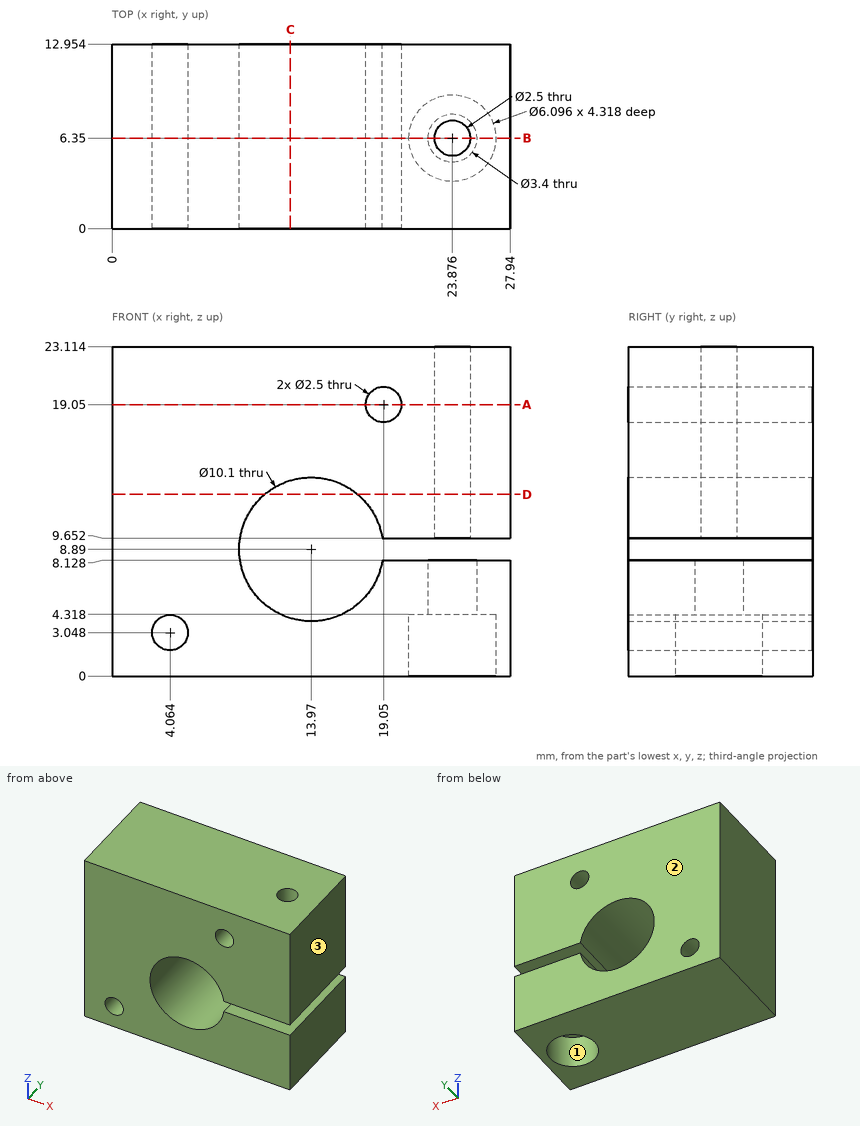
Geometry check sheet. Reference: drawing and pictorial views, mm from the part's lowest x, y, z. Coordinates: 2 decimals unless noted, no trailing zeros. Order: outer loops, then holes, each group sorted by start corner. A loop starts at its lowest first (then second) coordinate and runs counter-clockwise, first axis right, second up.
Item 1: Release check for a two-part mould opening along X. For the marked faces 1, 2 and 3 record: +X half, -X half, draft (parallel to the pull), parting line (faces both ways), or undercut.
Filled in:
face 1: undercut
face 2: draft
face 3: +X half
Item 2: Section check D-D, the plane z = 12.75. Enter the section's corners in (x, y).
Filled in:
outline: (0, 0) - (10.71, 0) - (10.71, 12.95) - (0, 12.95) - close; (17.23, 0) - (27.94, 0) - (27.94, 12.95) - (17.23, 12.95) - close; hole circle Ø2.5 at (23.88, 6.35)
Item 3: Material ranges on L1, parallel to Z at x = 20, y = 7.5; L2, parallel to Z at x = 22.75, y = 9.5; L3, parallel to X at y = 5.5, z = 18.75, recorded low to high.
Filled in:
L1: z = 0 to 8.13, 9.65 to 18.24, 19.86 to 23.11
L2: z = 0 to 8.13, 9.65 to 23.11
L3: x = 0 to 17.84, 20.26 to 22.96, 24.79 to 27.94
Item 4: Section check C-C, the plane x = 12.5. Enter the section's corners in (y, z).
Filled in:
outline: (0, 0) - (12.95, 0) - (12.95, 4.06) - (0, 4.06) - close; (0, 13.72) - (12.95, 13.72) - (12.95, 23.11) - (0, 23.11) - close
Item 5: Section check A-A, the plane z = 19.05. Enter the section's corners in (x, y).
Filled in:
outline: (0, 0) - (17.8, 0) - (17.8, 12.95) - (0, 12.95) - close; (20.3, 0) - (27.94, 0) - (27.94, 12.95) - (20.3, 12.95) - close; hole circle Ø2.5 at (23.88, 6.35)
Item 6: Depth check by flat-ended pin: pin 1 (3 mm diameter, centred on x = 23.876, y = 6.35, fed in from -Z); pin 2 (1.5 mm diameter, centred on x = 19.05, z = 19.05, fed in from -Y). Enter the tip coordinate at first touch or a pass-through.
Filled in:
pin 1: stops at z = 9.65
pin 2: passes through
Item 7: Section check B-B, the plane y = 6.35. Enter the section's corners in (x, z).
Filled in:
outline: (0, 0) - (20.83, 0) - (20.83, 4.32) - (22.18, 4.32) - (22.18, 8.13) - (18.96, 8.13) arc R5.05 cw (long way) to (18.96, 9.65) - (22.63, 9.65) - (22.63, 23.11) - (0, 23.11) - close; (25.13, 9.65) - (27.94, 9.65) - (27.94, 23.11) - (25.13, 23.11) - close; (25.58, 4.32) - (26.92, 4.32) - (26.92, 0) - (27.94, 0) - (27.94, 8.13) - (25.58, 8.13) - close; hole circle Ø2.5 at (4.06, 3.05); hole circle Ø2.5 at (19.05, 19.05)
